from build123d import *

# Parameters (mm, degrees)
SALIENTE_EXTRUIR1_DEPTH                = 45.6
CORTAR_EXTRUIR1_START                  = -37.6
CORTAR_EXTRUIR1_DEPTH                  = 37.6
CORTAR_EXTRUIR2_DEPTH                  = 37.6
SALIENTE_EXTRUIR2_DEPTH                = 10
CROQUIS5_W                             = 30.8
CROQUIS5_H                             = 10
CORTAR_EXTRUIR3_DEPTH                  = 118.087897795
CORTAR_EXTRUIR4_DEPTH                  = 3
CORTAR_EXTRUIR5_DEPTH                  = 3
CROQUIS8_W                             = 1.5
CROQUIS8_H                             = 35.841669751
DI_METRO_DE_TALADRO_3_0_3_1_AT_2_COUNT = 2
DI_METRO_DE_TALADRO_3_0_3_1_AT_2_PITCH = 20
DI_METRO_DE_TALADRO_3_0_3_2_D          = 3
DI_METRO_DE_TALADRO_3_0_3_2_DEPTH      = 4
DI_METRO_DE_TALADRO_3_2_3_2_1_D        = 3.2
DI_METRO_DE_TALADRO_3_2_3_2_1_DEPTH    = 4
DI_METRO_DE_TALADRO_3_0_3_3_D          = 3
DI_METRO_DE_TALADRO_3_0_3_3_DEPTH      = 4
DI_METRO_DE_TALADRO_3_0_3_4_D          = 3
DI_METRO_DE_TALADRO_3_0_3_5_D          = 3
DI_METRO_DE_TALADRO_3_0_3_5_DEPTH      = 45.6
DI_METRO_DE_TALADRO_3_2_3_2_2_D        = 3.2
DI_METRO_DE_TALADRO_3_2_3_2_2_DEPTH    = 4
DI_METRO_DE_TALADRO_3_2_3_2_3_D        = 3.2
DI_METRO_DE_TALADRO_3_2_3_2_4_D        = 3.2
DI_METRO_DE_TALADRO_3_2_3_2_4_DEPTH    = 45.6
DI_METRO_DE_TALADRO_3_0_3_6_D          = 3
DI_METRO_DE_TALADRO_3_0_3_6_DEPTH      = 71.241669751
REDONDEO1_R                            = 10


with BuildPart() as part:
    # Croquis1 → Saliente-Extruir1 (new body)
    with BuildSketch(Plane.XZ.offset(45.6)):
        with BuildLine():
            Line((65.468167059, 45.47114317), (17.015172443, 45.47114317))
            ThreePointArc((17.015172443, 45.47114317), (12.015172443, 44.131397208), (8.354918405, 40.47114317))
            Line((8.354918405, 40.47114317), (-6.258330249, 15.160254038))
            Line((-6.258330249, 15.160254038), (-3.660254038, 13.660254038))
            Line((-3.660254038, 13.660254038), (-8.660254038, 5))
            ThreePointArc((-8.660254038, 5), (-5, -8.660254038), (8.660254038, -5))
            Line((8.660254038, -5), (13.660254038, 3.660254038))
            Line((13.660254038, 3.660254038), (16.258330249, 2.160254038))
            Line((16.258330249, 2.160254038), (26.25277675, 19.47114317))
            Line((26.25277675, 19.47114317), (56.230562752, 19.47114317))
            Line((56.230562752, 19.47114317), (66.225009252, 2.160254038))
            Line((66.225009252, 2.160254038), (68.823085464, 3.660254038))
            Line((68.823085464, 3.660254038), (73.823085464, -5))
            ThreePointArc((73.823085464, -5), (87.483339502, -8.660254038), (91.143593539, 5))
            Line((91.143593539, 5), (86.143593539, 13.660254038))
            Line((86.143593539, 13.660254038), (88.741669751, 15.160254038))
            Line((88.741669751, 15.160254038), (74.128421097, 40.47114317))
            ThreePointArc((74.128421097, 40.47114317), (70.468167059, 44.131397208), (65.468167059, 45.47114317))
        make_face()
    extrude(amount=-SALIENTE_EXTRUIR1_DEPTH)

    # Croquis2 → Cortar-Extruir1 (cut)
    with BuildSketch(Plane(origin=(0, -4, 0), x_dir=(1, 0, 0), z_dir=(0, 1, 0)).offset(CORTAR_EXTRUIR1_START)):
        with BuildLine():
            Line((64.241669751, -45.47114317), (65.468167059, -45.47114317))
            ThreePointArc((65.468167059, -45.47114317), (70.468167059, -44.131397208), (74.128421097, -40.47114317))
            Line((74.128421097, -40.47114317), (88.741669751, -15.160254038))
            Line((88.741669751, -15.160254038), (86.143593539, -13.660254038))
            Line((86.143593539, -13.660254038), (91.143593539, -5))
            ThreePointArc((91.143593539, -5), (87.483339502, 8.660254038), (73.823085464, 5))
            Line((73.823085464, 5), (68.823085464, -3.660254038))
            Line((68.823085464, -3.660254038), (66.225009252, -2.160254038))
            Line((66.225009252, -2.160254038), (64.241669751, -5.595498823))
            Line((64.241669751, -5.595498823), (64.241669751, -45.47114317))
        make_face()
    extrude(amount=CORTAR_EXTRUIR1_DEPTH, mode=Mode.SUBTRACT)

    # Croquis3 → Cortar-Extruir2 (cut)
    with BuildSketch(Plane.XZ.offset(41.6)):
        with BuildLine():
            Line((18.241669751, 5.595498823), (18.241669751, 45.47114317))
            Line((18.241669751, 45.47114317), (17.015172443, 45.47114317))
            ThreePointArc((17.015172443, 45.47114317), (12.015172443, 44.131397208), (8.354918405, 40.47114317))
            Line((8.354918405, 40.47114317), (-6.258330249, 15.160254038))
            Line((-6.258330249, 15.160254038), (-3.660254038, 13.660254038))
            Line((-3.660254038, 13.660254038), (-8.660254038, 5))
            ThreePointArc((-8.660254038, 5), (-5, -8.660254038), (8.660254038, -5))
            Line((8.660254038, -5), (13.660254038, 3.660254038))
            Line((13.660254038, 3.660254038), (16.258330249, 2.160254038))
            Line((16.258330249, 2.160254038), (18.241669751, 5.595498823))
        make_face()
    extrude(amount=-CORTAR_EXTRUIR2_DEPTH, mode=Mode.SUBTRACT)

    # Croquis4 → Saliente-Extruir2 (add)
    with BuildSketch(Plane.XY.offset(45.47114317)):
        Polygon((65.468167059, -45.6), (17.015172443, -45.6), (17.015172443, -41.6), (18.241669751, -41.6), (18.241669751, -4), (17.015172443, -4), (17.015172443, 0), (65.468167059, 0), (65.468167059, -4), (64.241669751, -4), (64.241669751, -41.6), (65.468167059, -41.6), align=None)
    extrude(amount=SALIENTE_EXTRUIR2_DEPTH)

    # Croquis5 → Cortar-Extruir3 (cut, through all)
    with BuildSketch(Plane(origin=(0, 0, 0), x_dir=(-1, 0, 0), z_dir=(0, 1, 0))):
        with Locations((-41.241669751, 50.47114317)):
            Rectangle(CROQUIS5_W, CROQUIS5_H)
    extrude(amount=-CORTAR_EXTRUIR3_DEPTH, mode=Mode.SUBTRACT)

    # Croquis6 → Cortar-Extruir4 (cut)
    with BuildSketch(Plane(origin=(64.241669751, 0, 0), x_dir=(0, 0, -1), z_dir=(1, 0, 0))):
        Polygon((-47.620680834, -34.444647218), (-47.621605732, -31.153750813), (-50.472068068, -29.509103596), (-53.321605506, -31.155352782), (-53.320680609, -34.446249187), (-50.470218273, -36.090896404), align=None)
    extrude(amount=-CORTAR_EXTRUIR4_DEPTH, mode=Mode.SUBTRACT)

    # Croquis7 → Cortar-Extruir5 (cut)
    with BuildSketch(Plane(origin=(64.241669751, 0, 0), x_dir=(0, 0, -1), z_dir=(1, 0, 0))):
        Polygon((-50.470218273, -9.509103596), (-53.320680609, -11.153750813), (-53.321605506, -14.444647218), (-50.472068068, -16.090896404), (-47.621605732, -14.446249187), (-47.620680834, -11.155352782), align=None)
    extrude(amount=-CORTAR_EXTRUIR5_DEPTH, mode=Mode.SUBTRACT)

    # Croquis8 → Diámetro de taladro Ø3.0 (3)1 (revolve, cut)
    with BuildSketch(Plane(origin=(25.841669751, -12.8, 50.47114317), x_dir=(0, 0, -1), z_dir=(0, 1, 0))):
        with Locations((0.75, 17.920834876)):
            Rectangle(CROQUIS8_W, CROQUIS8_H)
    di_metro_de_taladro_3_0_3_1 = revolve(axis=Axis((32.191669751, -12.8, 50.47114317), (-1, 0, 0)), mode=Mode.SUBTRACT)

    # Diámetro de taladro Ø3.0 (3)1 at 2: Diámetro de taladro Ø3.0 (3)1 ×2
    with Locations(*[(0, -i * DI_METRO_DE_TALADRO_3_0_3_1_AT_2_PITCH, 0) for i in range(1, DI_METRO_DE_TALADRO_3_0_3_1_AT_2_COUNT)]):
        add(di_metro_de_taladro_3_0_3_1, mode=Mode.SUBTRACT)

    # Diámetro de taladro Ø3.0 (3)2
    with Locations(Plane(origin=(0, -45.6, 0), x_dir=(-1, 0, 0), z_dir=(0, -1, 0))):
        with Locations((-89.483339502, 0), (-75.483339502, 0)):
            Hole(DI_METRO_DE_TALADRO_3_0_3_2_D / 2, depth=DI_METRO_DE_TALADRO_3_0_3_2_DEPTH)

    # Diámetro de taladro Ø3.2 (3.2)1
    with Locations(Plane(origin=(0, -45.6, 0), x_dir=(-1, 0, 0), z_dir=(0, -1, 0))):
        with Locations((-82.483339502, 0)):
            Hole(DI_METRO_DE_TALADRO_3_2_3_2_1_D / 2, depth=DI_METRO_DE_TALADRO_3_2_3_2_1_DEPTH)

    # Diámetro de taladro Ø3.0 (3)3
    with Locations(Plane(origin=(0, -4, 0), x_dir=(-1, 0, 0), z_dir=(0, -1, 0))):
        with Locations((-7, 0), (7, 0)):
            Hole(DI_METRO_DE_TALADRO_3_0_3_3_D / 2, depth=DI_METRO_DE_TALADRO_3_0_3_3_DEPTH)

    # Diámetro de taladro Ø3.0 (3)4 (through all)
    with Locations(Plane(origin=(0, -41.6, 0), x_dir=(1, 0, 0), z_dir=(0, 1, 0))):
        with Locations((7, 0), (-7, 0)):
            Hole(DI_METRO_DE_TALADRO_3_0_3_4_D / 2)

    # Diámetro de taladro Ø3.0 (3)5
    with Locations(Plane(origin=(0, 0, 0), x_dir=(1, 0, 0), z_dir=(0, 1, 0))):
        with Locations((89.483339502, 0), (75.483339502, 0)):
            Hole(DI_METRO_DE_TALADRO_3_0_3_5_D / 2, depth=DI_METRO_DE_TALADRO_3_0_3_5_DEPTH)

    # Diámetro de taladro Ø3.2 (3.2)2
    with Locations(Plane(origin=(0, -4, 0), x_dir=(-1, 0, 0), z_dir=(0, -1, 0))):
        with Locations((0, 0)):
            Hole(DI_METRO_DE_TALADRO_3_2_3_2_2_D / 2, depth=DI_METRO_DE_TALADRO_3_2_3_2_2_DEPTH)

    # Diámetro de taladro Ø3.2 (3.2)3 (through all)
    with Locations(Plane(origin=(0, -41.6, 0), x_dir=(1, 0, 0), z_dir=(0, 1, 0))):
        with Locations((0, 0)):
            Hole(DI_METRO_DE_TALADRO_3_2_3_2_3_D / 2)

    # Diámetro de taladro Ø3.2 (3.2)4
    with Locations(Plane(origin=(0, 0, 0), x_dir=(1, 0, 0), z_dir=(0, 1, 0))):
        with Locations((82.483339502, 0)):
            Hole(DI_METRO_DE_TALADRO_3_2_3_2_4_D / 2, depth=DI_METRO_DE_TALADRO_3_2_3_2_4_DEPTH)

    # Diámetro de taladro Ø3.0 (3)6
    with Locations(Plane(origin=(61.241669751, 0, 0), x_dir=(0, 0, -1), z_dir=(1, 0, 0))):
        with Locations((-50.47114317, -12.8), (-50.47114317, -32.8)):
            Hole(DI_METRO_DE_TALADRO_3_0_3_6_D / 2, depth=DI_METRO_DE_TALADRO_3_0_3_6_DEPTH)

    # Redondeo1
    redondeo1_edges = [part.edges().sort_by_distance(p)[0] for p in [
        (56.230562752, -22.8, 19.47114317),
        (26.25277675, -22.8, 19.47114317),
    ]]
    fillet(redondeo1_edges, radius=REDONDEO1_R)


solid = part.part
Design review of the part built by this model. Coordinates are the model's own, in mm. A direction names the side the tool comes from. Round coordinates to 2 decimals unless told otherwise and drop trailing zeros. Loops run counter-clockwise (first coordinate to the right, second up) from the corner with the lowest first, then second, coordinate; pieces in that order, holes last. Notation, with made-up numbers: (3.25, 10) - (14.25, 10) arc R24 cw to (14.25, 42) - close; hole circle Ø8 at (-13.75, 82.5). An arc over 180 degrees is marked (long way). One line per item, written item: value. Start each with the question number.
1) To check wall thickness, follow L1, parallel to Y at x = 82, z = 16; L2, parallel to X at y = -33, z = 46; L3, parallel to Z at x = 50, y = -25. State the ranges of each line that lie inside material, in increasing order. Write a range as from..to.
2) Insertion check: pin 1 Ø4 at (y, z) = (-12.8, 50.47) entering from +X; pin 2 Ø12 at (y, z) = (-14, 0) entering from -X; pin 3 Ø3 at (y, z) = (-43.5, 50.5) entering from +X. Each pin has a flat end and moves straight along its axis. Give the tip position at first contact, or say it passes through.
3) Consider section D-D on z = 21.5. Give the boundary of the cut face in (x, y).
4) Consider section B-B on y = -12.8. Give the boundary of the cut face in (x, z), then the cut area to 3 significant figures.
5) Draft analysis for pull direction Z (two halves, no side actions). For faces 5 (the flat face through (61, -22, 55.471)), 6 (the cylindrical face through (1.27, -43.63, 0.97)), 7 (the cylindrical face through (87.29, -43.63, -8.77)), state which applies: +Z half, -Z half, draft (parallel to the pull), parting line (faces both ways), or undercut.
6) Consider section C-C on y = -38.5. Give the boundary of the cut face in (x, z), then the cut area to 3 significant figures.
7) Consider section A-A on x = 0. Give the boundary of the cut face in (y, z), then the cut area to 3 significant figures.
8) For faces 1 (the flat face through (67.51, -43.63, 2.9)), 2 (the flat face through (62.763, -30.321, 51.877)), 3 (the flat face through (75, -41.6, 15)), 4 (the flat face through (25.842, -22, 50)), list the 3-axis set-ups (+Z, -Z, +X, -X, +Y, -Y) from which the entire face can be reached by the end or side of a thin tool; tool diameter is ignored.
Reported:
1. L1: y = -45.6..-41.6, -4..0
1. L2: x = 18.24..25.84, 56.64..64.24
1. L3: z = 19.47..45.47
2. pin 1: stops at x = 61.24
2. pin 2: stops at x = 18.24
2. pin 3: stops at x = 65.47
3. outline: (-2.6, -45.6) - (85.08, -45.6) - (85.08, -41.6) - (64.24, -41.6) - (64.24, -4) - (85.08, -4) - (85.08, 0) - (-2.6, 0) - (-2.6, -4) - (18.24, -4) - (18.24, -41.6) - (-2.6, -41.6) - close
4. outline: (18.24, 5.6) - (23.37, 14.47) arc R10 cw to (32.03, 19.47) - (50.46, 19.47) arc R10 cw to (59.12, 14.47) - (64.24, 5.6) - (64.24, 47.62) - (61.24, 47.62) - (61.24, 48.97) - (56.64, 48.97) - (56.64, 45.47) - (25.84, 45.47) - (25.84, 48.97) - (18.24, 48.97) - close; (18.24, 51.97) - (25.84, 51.97) - (25.84, 55.47) - (18.24, 55.47) - close; (56.64, 51.97) - (61.24, 51.97) - (61.24, 53.32) - (64.24, 53.32) - (64.24, 55.47) - (56.64, 55.47) - close
4. area: 1,420 mm^2
5. face 5: +Z half
5. face 6: undercut
5. face 7: parting line
6. outline: (18.24, 5.6) - (23.37, 14.47) arc R10 cw to (32.03, 19.47) - (50.46, 19.47) arc R10 cw to (59.12, 14.47) - (64.24, 5.6) - (64.24, 55.47) - (56.64, 55.47) - (56.64, 45.47) - (25.84, 45.47) - (25.84, 55.47) - (18.24, 55.47) - close
6. area: 1,470 mm^2
7. outline: (-45.6, -10) - (-41.6, -10) - (-41.6, -1.6) - (-45.6, -1.6) - close; (-45.6, 1.6) - (-41.6, 1.6) - (-41.6, 26) - (-45.6, 26) - close; (-4, -10) - (0, -10) - (0, -1.6) - (-4, -1.6) - close; (-4, 1.6) - (0, 1.6) - (0, 26) - (-4, 26) - close
7. area: 262 mm^2
8. face 1: -Z, +Y, -Y
8. face 2: +X
8. face 3: +Z, -Z, +X
8. face 4: +Z, +Y, -Y
